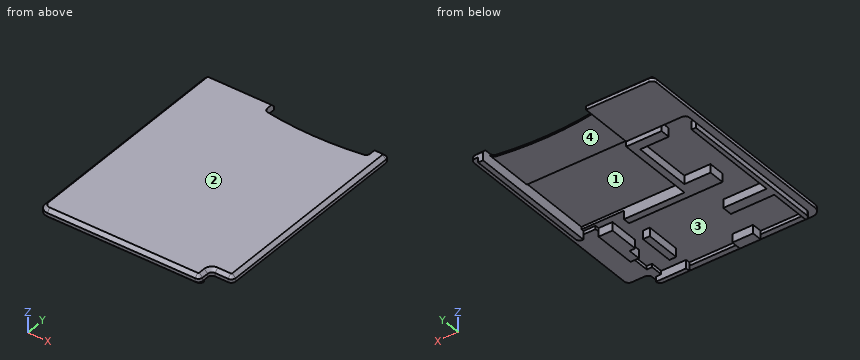
```python
from build123d import *

# Parameters (mm, degrees)
SKIZZE2_W                                   = 21.5
SKIZZE2_H                                   = 26.5
AUFSATZ_LINEAR_AUSTRAGEN1_DEPTH             = 0.8
AUFSATZ_LINEAR_AUSTRAGEN2_DEPTH             = 0.6
SCHNITT_LINEAR_AUSTRAGEN2_DEPTH             = 0.7
SCHNITT_LINEAR_AUSTRAGEN2_DEPTH_BACK        = 40.270886163
SKIZZE5_W                                   = 12.144981168
SKIZZE5_H                                   = 8.613973721
SCHNITT_LINEAR_AUSTRAGEN1_DEPTH             = 0.4
SCHNITT_LINEAR_AUSTRAGEN1_DEPTH_BACK        = 40.270886163
SCHNITT_LINEAR_AUSTRAGEN3_DEPTH             = 0.6
SCHNITT_LINEAR_AUSTRAGEN3_DEPTH_BACK        = 40.270886163
SKIZZE6_W                                   = 12.144981168
SKIZZE6_H                                   = 8.023619308
VERRUNDUNG1_R                               = 0.5
SCHNITT_LINEAR_AUSTRAGEN4_DEPTH             = 40.270886163
SCHNITT_LINEAR_AUSTRAGEN4_DEPTH_BACK        = 40.270886163
VERRUNDUNG3_R                               = 0.5
SKIZZE8_W                                   = 5.461913831
SKIZZE8_H                                   = 1.2
SKIZZE8_W_2                                 = 0.8
SKIZZE8_H_2                                 = 4.167109648
AUFSATZ_LINEAR_AUSTRAGEN3_DEPTH             = 0.6
AUFSATZ_LINEAR_AUSTRAGEN3_DIRECTION_2_REACH = 41.271
SCHNITT_LINEAR_AUSTRAGEN5_DEPTH             = 40.270886163
SCHNITT_LINEAR_AUSTRAGEN5_DEPTH_BACK        = 40.270886163
SKIZZE9_W                                   = 2.954983754
SKIZZE9_H                                   = 2.164950306
SKIZZE10_W                                  = 0.770433568
SKIZZE10_H                                  = 2.170677495
AUFSATZ_LINEAR_AUSTRAGEN4_DEPTH             = 0.8
VERRUNDUNG2_R                               = 1
VERRUNDUNG4_R                               = 0.5
FASE1_SIZE                                  = 0.4


with BuildPart() as part:
    # Skizze2 → Aufsatz-Linear austragen1 (new body)
    with BuildSketch(Plane.XY.offset(1.2)):
        with Locations((12, 18.75)):
            Rectangle(SKIZZE2_W, SKIZZE2_H)
    extrude(amount=AUFSATZ_LINEAR_AUSTRAGEN1_DEPTH)

    # Skizze3 → Aufsatz-Linear austragen2 (add)
    with BuildSketch(Plane.XY.offset(1.2)):
        Polygon((21.9, 32), (21.9, 16.15), (19.9, 16.15), (19.9, 6.15), (2.1, 6.15), (2.1, 25.65), (10, 25.65), (10, 32), align=None)
    extrude(amount=-AUFSATZ_LINEAR_AUSTRAGEN2_DEPTH)

    # Skizze5 → Schnitt-Linear austragen2 (cut, two sides: drawn at the far end of the back side and taken through both)
    with BuildSketch(Plane.XY.offset(1.2).offset(-SCHNITT_LINEAR_AUSTRAGEN2_DEPTH_BACK)):
        with Locations((15.254893919, 20.77736777)):
            Rectangle(SKIZZE5_W, SKIZZE5_H)
    extrude(amount=SCHNITT_LINEAR_AUSTRAGEN2_DEPTH + SCHNITT_LINEAR_AUSTRAGEN2_DEPTH_BACK, mode=Mode.SUBTRACT)

    # Skizze4 → Schnitt-Linear austragen1 (cut, two sides: drawn at the far end of the back side and taken through both)
    with BuildSketch(Plane.XY.offset(1.2).offset(-SCHNITT_LINEAR_AUSTRAGEN1_DEPTH_BACK)):
        Polygon((8.382403335, 24.511668734), (5.015709698, 24.511668734), (5.015709698, 25.65), (2.1, 25.65), (2.1, 24.134887808), (2.6, 24.134887808), (2.6, 6.15), (7.902667193, 6.15), (7.902667193, 7.35), (10.352191741, 7.35), (10.352191741, 6.15), (16.321024544, 6.15), (16.321024544, 6.65), (19.9, 6.65), (19.9, 10.624393956), (18.922805677, 10.624393956), (18.922805677, 12.094523693), (18.263327803, 12.094523693), (18.263327803, 15.67038091), (19.9, 15.67038091), (19.9, 16.15), (21.327384503, 16.15), (21.327384503, 16.47038091), (16.321024544, 16.47038091), (16.321024544, 15.67038091), (5.294026876, 15.67038091), (5.294026876, 17.554984477), (8.382403335, 17.554984477), align=None)
    extrude(amount=SCHNITT_LINEAR_AUSTRAGEN1_DEPTH + SCHNITT_LINEAR_AUSTRAGEN1_DEPTH_BACK, mode=Mode.SUBTRACT)

    # Skizze6 → Schnitt-Linear austragen3 (cut, two sides: drawn at the far end of the back side and taken through both)
    with BuildSketch(Plane.XY.offset(1.2).offset(-SCHNITT_LINEAR_AUSTRAGEN3_DEPTH_BACK)):
        with Locations((15.254893919, 29.096164285)):
            Rectangle(SKIZZE6_W, SKIZZE6_H)
    extrude(amount=SCHNITT_LINEAR_AUSTRAGEN3_DEPTH + SCHNITT_LINEAR_AUSTRAGEN3_DEPTH_BACK, mode=Mode.SUBTRACT)

    # Verrundung1
    verrundung1_edges = [part.edges().sort_by_distance(p)[0] for p in [
        (21.9, 16.15, 0.9),
        (2.1, 25.65, 1.4),
        (2.1, 6.15, 0.9),
        (19.9, 6.15, 0.9),
    ]]
    fillet(verrundung1_edges, radius=VERRUNDUNG1_R - 0.0001)  # a hair under: the kernel refuses the full size

    # Skizze7 → Schnitt-Linear austragen4 (cut, two sides: drawn at the far end of the back side and taken through both)
    with BuildSketch(Plane.XY.offset(1.2).offset(-SCHNITT_LINEAR_AUSTRAGEN4_DEPTH_BACK)):
        with BuildLine():
            Line((21.327384503, 30.5), (21.327384503, 32.799881912))
            Line((21.327384503, 32.799881912), (9.182403335, 32.799881912))
            Line((9.182403335, 32.799881912), (9.182403335, 30.5))
            ThreePointArc((9.182403335, 30.5), (15.254893919, 30), (21.327384503, 30.5))
        make_face()
    extrude(amount=SCHNITT_LINEAR_AUSTRAGEN4_DEPTH + SCHNITT_LINEAR_AUSTRAGEN4_DEPTH_BACK, mode=Mode.SUBTRACT)

    # Verrundung3
    verrundung3_edges = [part.edges().sort_by_distance(p)[0] for p in [
        (9.182403335, 30.5, 1.9),
        (21.327384503, 30.5, 1.9),
    ]]
    fillet(verrundung3_edges, radius=VERRUNDUNG3_R)

    # Skizze8 → Aufsatz-Linear austragen3 (add)
    with BuildSketch(Plane.XY.offset(1.2)):
        with Locations((4.988422265, 11.700335539)):
            Rectangle(SKIZZE8_W, SKIZZE8_H)
        with Locations((16.376411907, 10.759758473)):
            Rectangle(SKIZZE8_W_2, SKIZZE8_H_2)
    extrude(amount=-AUFSATZ_LINEAR_AUSTRAGEN3_DEPTH)

    # Skizze8 → Aufsatz-Linear austragen3 direction 2 (add, up to next)
    with BuildSketch(Plane.XY.offset(1.2), mode=Mode.PRIVATE) as aufsatz_linear_austragen3_direction_2_sk1:
        with Locations((4.988422265, 11.700335539)):
            Rectangle(SKIZZE8_W, SKIZZE8_H)
    aufsatz_linear_austragen3_direction_2_tool1 = extrude(aufsatz_linear_austragen3_direction_2_sk1.sketch, amount=AUFSATZ_LINEAR_AUSTRAGEN3_DIRECTION_2_REACH, mode=Mode.PRIVATE) - part.part
    # Skizze8 → Aufsatz-Linear austragen3 direction 2 (add, up to next)
    with BuildSketch(Plane.XY.offset(1.2), mode=Mode.PRIVATE) as aufsatz_linear_austragen3_direction_2_sk2:
        with Locations((16.376411907, 10.759758473)):
            Rectangle(SKIZZE8_W_2, SKIZZE8_H_2)
    aufsatz_linear_austragen3_direction_2_tool2 = extrude(aufsatz_linear_austragen3_direction_2_sk2.sketch, amount=AUFSATZ_LINEAR_AUSTRAGEN3_DIRECTION_2_REACH, mode=Mode.PRIVATE) - part.part
    add(aufsatz_linear_austragen3_direction_2_tool1.solids().sort_by_distance((4.988422, 11.700336, 1.2))[0])
    add(aufsatz_linear_austragen3_direction_2_tool2.solids().sort_by_distance((16.376412, 10.759758, 1.2))[0])

    # Skizze9 → Schnitt-Linear austragen5 (cut, two sides: drawn at the far end of the back side and taken through both)
    with BuildSketch(Plane.XY.offset(1.2).offset(-SCHNITT_LINEAR_AUSTRAGEN5_DEPTH_BACK)):
        with Locations((21.677491877, 6.217524847)):
            Rectangle(SKIZZE9_W, SKIZZE9_H)
    extrude(amount=SCHNITT_LINEAR_AUSTRAGEN5_DEPTH + SCHNITT_LINEAR_AUSTRAGEN5_DEPTH_BACK, mode=Mode.SUBTRACT)

    # Skizze10 → Aufsatz-Linear austragen4 (add)
    with BuildSketch(Plane.XY.offset(1.2)):
        with Locations((19.652022519, 6.998720979)):
            Rectangle(SKIZZE10_W, SKIZZE10_H)
    extrude(amount=AUFSATZ_LINEAR_AUSTRAGEN4_DEPTH)

    # Verrundung2
    verrundung2_edges = [part.edges().sort_by_distance(p)[0] for p in [
        (1.25, 5.5, 1.6),
    ]]
    fillet(verrundung2_edges, radius=VERRUNDUNG2_R)

    # Verrundung4
    verrundung4_edges = [part.edges().sort_by_distance(p)[0] for p in [
        (22.75, 7.3, 1.6),
        (20.2, 5.5, 1.6),
        (20.2, 7.3, 1.6),
        (1.25, 32, 1.6),
        (22.75, 32, 1.6),
    ]]
    fillet(verrundung4_edges, radius=VERRUNDUNG4_R)

    # Fase1
    fase1_edges = [part.edges().sort_by_distance(p)[0] for p in [
        (5.466201668, 32, 2),
        (10.975, 5.5, 2),
        (1.542893219, 5.792893219, 2),
        (22.75, 19.65, 2),
        (21.475, 7.3, 2),
        (1.25, 19, 2),
        (20.2, 6.4, 2),
        (21.788692251, 32, 2),
        (1.396446609, 31.853553391, 2),
        (22.603553391, 31.853553391, 2),
        (20.053553391, 5.646446609, 2),
        (22.603553391, 7.446446609, 2),
        (20.346446609, 7.153553391, 2),
    ]]
    chamfer(fase1_edges, length=FASE1_SIZE)


solid = part.part
```
Here's how the part is built. I have some questions about the finished solid (model axes, mm). Face numbers are marked on the shaded views. A direction names the side the tool comes from. Give positions to 0.01 mm unless a question says otherwise; leave off trailing zeros. Write each loop counter-clockwise with the first axis right and the second up, starting at its lowest first coordinate (ties: lowest second). Pieces come first, ordered by that corner, then holes.
(1) If I drill on L1, parallel to Y at x = 7, z = 1.05; L2, parallel to X at y = 12.25, z = 1.05; L3, parallel to Y at x = 16.25, z = 1.3, over which ranges is the centre line in solid material (lowest first)?
Output values:
L1: y = 11.1 to 12.3, 15.67 to 17.55, 24.51 to 25.65
L2: x = 2.1 to 7.72, 15.98 to 16.78, 18.26 to 19.9
L3: y = 5.5 to 6.15, 8.68 to 12.84, 15.67 to 16.47
(2) Imagine slicing it at A-A, the plane y = 11.75. Write out the boundary of the cut face in (x, z).
Output values:
outline: (1.25, 1.2) - (2.1, 1.2) - (2.1, 0.6) - (7.72, 0.6) - (7.72, 1.6) - (15.98, 1.6) - (15.98, 0.6) - (16.78, 0.6) - (16.78, 1.6) - (18.92, 1.6) - (18.92, 0.6) - (19.9, 0.6) - (19.9, 1.2) - (22.75, 1.2) - (22.75, 1.6) - (22.35, 2) - (1.65, 2) - (1.25, 1.6) - close
(3) Imagine slicing it at B-B, the plane z = 0.95. Count the separate pieces of the cut face and the enclosed holes in it, and give its area (4 significant figures).
Output values:
separate pieces: 7
enclosed holes: 0
area: 62.75 mm2
(4) Thinking about a two-plate mould opening in Y: for the marked faces 3 and 4, which applies, pulls with the +Y half, pulls with the -Y half, needs draft (parallel to the pull), parting line crosses it, or undercut?
Output values:
face 3: undercut
face 4: needs draft
(5) Imagine slicing it at D-D, the plane y = 9. Write out the boundary of the cut face in (x, z).
Output values:
outline: (1.25, 1.2) - (2.1, 1.2) - (2.1, 0.6) - (2.6, 0.6) - (2.6, 1.6) - (15.98, 1.6) - (15.98, 0.6) - (16.78, 0.6) - (16.78, 1.6) - (19.9, 1.6) - (19.9, 1.2) - (22.75, 1.2) - (22.75, 1.6) - (22.35, 2) - (1.65, 2) - (1.25, 1.6) - close
(6) On a 3-axis mill with a long thin cutter (end or side, diameter ignored), from which of +Z, -Z, +X, -X, +Y, -Y can I reach the whole of each face in a straight line? I mean the marked faces 1 and 2. Say none if no direction works.
Output values:
face 1: -Z
face 2: +Z, +X, -X, +Y, -Y
(7) Will this pin go through, and if not, where does the flat tip stop? pin 1 (0.8 mm diameter, centred on x = 19, z = 1, fed in from +Y).
Output values:
pin 1: stops at y = 15.67
(8) Imagine slicing it at C-C, the plane x = 6. Write out the boundary of the cut face in (y, z).
Output values:
outline: (5.5, 1.2) - (6.15, 1.2) - (6.15, 1.6) - (11.1, 1.6) - (11.1, 0.6) - (12.3, 0.6) - (12.3, 1.6) - (15.67, 1.6) - (15.67, 0.6) - (17.55, 0.6) - (17.55, 1.6) - (24.51, 1.6) - (24.51, 0.6) - (25.65, 0.6) - (25.65, 1.2) - (32, 1.2) - (32, 1.6) - (31.6, 2) - (5.9, 2) - (5.5, 1.6) - close
